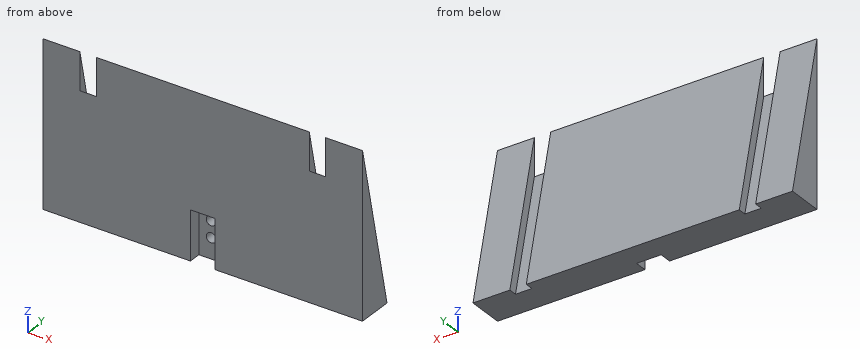
Autodesk Inventor part; units mm, degrees
ref_plane "YZ Plane" through (0, 0, 0) normal (1, 0, 0) x (0, 1, 0)
ref_plane "XZ Plane" through (0, 0, 0) normal (0, 1, 0) x (-1, 0, 0)
ref_plane "XY Plane" through (0, 0, 0) normal (0, 0, 1) x (1, 0, 0)
sketch "草图2" plane through (0, 0, 0) normal (1, 0, 0) x (0, 1, 0)
  line L0 (120, -550) -> (0, 0)
  line L1 (0, 0) -> (0, -550)
  line L2 (0, -550) -> (120, -550)
  line L3 (43.6364, -200) -> (0, -200)
  dimension "d0" = 120
  dimension "d1" = 550
  dimension "d2" = 200
extrude "拉伸1" add sketch "草图2" along normal mid plane 390 contours L3 L1 L0
sketch "草图3" plane through (-195, 0, 0) normal (0, 0.9770158, 0.2131671) x (1, 0, 0)
  line L0 (0, 0) -> (390, 0)
  line L1 (390, 204.705) -> (0, 204.705)
  line L2 (325, 0) -> (345, 0)
  line L3 (345, 0) -> (345, 204.705)
  line L4 (345, 204.705) -> (325, 204.705)
  line L5 (325, 204.705) -> (325, 0)
  line L6 (390, 204.705) -> (390, 0)
  point P0 (195, 0)
  dimension "d5" = 20
  dimension "d6" = 45
sketch "草图4" plane through (195, 43.6364, -200) normal (0, 0, -1) x (-1, 0, 0)
  line L0 (45, 0) -> (45, -10)
  point P0 (195, -43.6364)
  dimension "d8" = 10
sweep "扫掠1" cut profiles "草图3" path "草图4" contours L5 L1 L3 L0
mirror "镜像1" about plane through (0, 0, 0) normal (1, 0, 0) of "扫掠1"
sketch "草图5" plane through (-195, 0, -200) normal (0, -1, 0) x (1, 0, 0)
  line L0 (195, -50) -> (195, 300)
  line L1 (0, 0) -> (390, 0)
  line L2 (210, 0) -> (180, 0)
  line L3 (180, 0) -> (180, 60)
  line L4 (180, 60) -> (210, 60)
  line L5 (210, 60) -> (210, 0)
  point P0 (195, 200)
  point P1 (180, 0)
  dimension "d11" = 60
  dimension "d12" = 30
extrude "拉伸2" cut sketch "草图5" against normal blind 15
sketch "草图6" plane through (-195, 15, -200) normal (0, -1, 0) x (1, 0, 0)
  line L0 (210, 0) -> (180, 0)
  line L1 (180, 60) -> (210, 60)
  line L2 (180, 0) -> (180, 60)
  line L3 (210, 0) -> (180, 0)
  line L4 (210, 60) -> (210, 0)
  line L5 (195, -11.4626) -> (195, 50.2539)
  circle A0 centre (195, 25) radius 6
  circle A1 centre (195, 45) radius 6
  point P0 (195, 200)
  dimension "d15" = 30
  dimension "d16" = 12
  dimension "d17" = 12
  dimension "d18" = 20
  dimension "d19" = 25
extrude "拉伸3" cut sketch "草图6" against normal blind 15 contours A0 L5 | L5 A0 | A1
thread "螺纹1"
thread "螺纹2"
properties part number "猫砂盆底座"
The model under review builds one solid part; all positions refer to its coordinate system, in mm. Coordinates: 2 decimals unless noted, no trailing zeros. Write each loop counter-clockwise with the first axis right and the second up, starting at its lowest first coordinate (ties: lowest second). Pieces come first, ordered by that corner, then holes. Notation, with made-up numbers: (64, 4.25) -> (97, 4.25) arc R32 cw to (97, 32.25) -> close; hole circle Ø1 at (82.5, 59). An arc over 180 degrees is marked (long way). One line per item, written item: value. Start each with the question number.
Q1. To check wall thickness, follow probe 1 along X at (y, z) = (25, -155); probe 2 along X at (y, z) = (21.5, -99.5); probe 3 along X at (y, z) = (18.75, -175). State the ranges of each line that lie inside material, in increasing order.
Q2. Add section C-C, the plane x = 0. Give the boundary of the cut face in (y, z), then the cut area to 3 significant figures.
Q3. Clearance check with flat-ended pins moving along their axes: P1, Ø13, axis at x = -2.5, z = -176, coming from the -Y side; P2, Ø5, axis at x = -136, z = -176.5, coming from the +Y side; P3, Ø16.5, axis at x = -6, y = 4.5, coming from the -Z side. State where each tip first meets the part, or that it passes through.
Q4. Add section A-A, the plane y = 39. Give the boundary of the cut face in (x, z).
Q5. Add section D-D, the plane y = 9.5. Give the boundary of the cut face in (x, z).
Q6. Add section B-B, the plane z = -155. Give the boundary of the cut face in (x, y), then the cut area to 3 significant figures.
Response:
1. probe 1: -195 to -150, -130 to -6, 6 to 130, 150 to 195
1. probe 2: -195 to -150, -130 to 130, 150 to 195
1. probe 3: -195 to -6, 6 to 195
2. outline: (0, -140) -> (15, -140) -> (15, -149) -> (30, -149) -> (30, -161) -> (15, -161) -> (15, -169) -> (30, -169) -> (30, -181) -> (15, -181) -> (15, -200) -> (43.64, -200) -> (0, 0) -> close
2. area: 3,100 mm²
3. P1: y = 15
3. P2: y = 29.05
3. P3: z = -140
4. outline: (-195, -200) -> (-150, -200) -> (-150, -178.75) -> (-195, -178.75) -> close; (-130, -200) -> (130, -200) -> (130, -178.75) -> (-130, -178.75) -> close; (150, -200) -> (195, -200) -> (195, -178.75) -> (150, -178.75) -> close
5. outline: (-195, -200) -> (-15, -200) -> (-15, -140) -> (15, -140) -> (15, -200) -> (195, -200) -> (195, -43.54) -> (150, -43.54) -> (150, -89.37) -> (130, -89.37) -> (130, -43.54) -> (-130, -43.54) -> (-130, -89.37) -> (-150, -89.37) -> (-150, -43.54) -> (-195, -43.54) -> close
6. outline: (-195, 0) -> (-15, 0) -> (-15, 15) -> (-6, 15) -> (-6, 30) -> (6, 30) -> (6, 15) -> (15, 15) -> (15, 0) -> (195, 0) -> (195, 33.82) -> (150, 33.82) -> (150, 23.82) -> (130, 23.82) -> (130, 33.82) -> (-130, 33.82) -> (-130, 23.82) -> (-150, 23.82) -> (-150, 33.82) -> (-195, 33.82) -> close
6. area: 12,200 mm²
